Job drawing, mm, ordinate dimensions from the low corner. One solid piece. Round coordinates to 2 decimals unless told otherwise and drop trailing zeros. Order: outer loops, then holes, each group sorted by start corner. A loop starts at its lowest first (then second) coordinate and runs counter-clockwise, first axis right, second up. Notation, with made-up numbers: (55.5, -21.75) - (85.5, -21.75) arc R4 cw to (85.5, -14.75) - close; hole circle Ø5 at (78, 77.5). An arc over 180 degrees is marked (long way). Use one line per item in the form item = value. Start each with the question number.
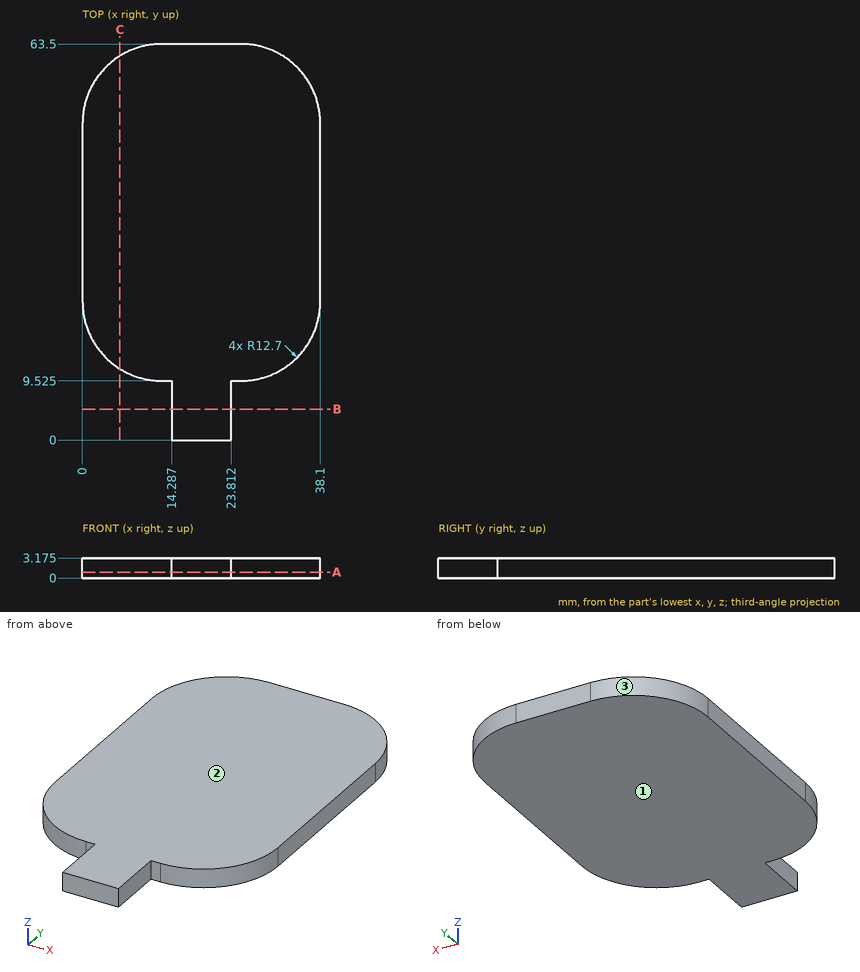
(1) Flat gauge pins, fed straight in: P1, Ø0.8, axis at x = 25, z = 2, coming from the -Y side (1 decimal); P2, Ø1, axis at y = 20.5, z = 1.5, coming from the +X side. Where does each tip first touch, or does it go through?
(2) Mould opens along Z. For the marked faces 1, 2 and 3 say: pulls with the +Z half, pulls with the -Z half, needs draft (parallel to the pull), parting line crosses it, or undercut.
(3) Slice it at B-B (y = 5). Give the cut face in (x, z) (1 decimal).
(4) Slice it at A-A (z = 0.95). Give the cut face in (x, y) (1 decimal), and give its area (3 significant figures).
(5) Slice it at C-C (x = 6). Give the cut face in (y, z) (1 decimal), and give its area (3 significant figures).
(6) Wall check: line 1 (X direction, y = 51, z = 2.75); line 2 (X direction, y = 7.5, z = 0.5); line 3 (Y direction, x = 14, z = 2.1) (1 decimal). Give the ranges that are in metal, low to high. Write a range as [from, to].
Results list:
q1.P1 = 9.5
q1.P2 = 38.04
q2.face_1 = pulls with the -Z half
q2.face_2 = pulls with the +Z half
q2.face_3 = needs draft
q3.outline = (14.3, 0) - (23.8, 0) - (23.8, 3.2) - (14.3, 3.2) - close
q4.outline = (0, 22.2) arc R12.7 ccw to (12.7, 9.5) - (14.3, 9.5) - (14.3, 0) - (23.8, 0) - (23.8, 9.5) - (25.4, 9.5) arc R12.7 ccw to (38.1, 22.2) - (38.1, 50.8) arc R12.7 ccw to (25.4, 63.5) - (12.7, 63.5) arc R12.7 ccw to (0, 50.8) - close
q4.area = 2,010 mm²
q5.outline = (11.4, 0) - (61.6, 0) - (61.6, 3.2) - (11.4, 3.2) - close
q5.area = 159 mm²
q6.line_1 = [0, 38.1]
q6.line_2 = [14.29, 23.81]
q6.line_3 = [9.5, 63.5]
